The model under review builds one solid part; all positions refer to its coordinate system, in mm. Face numbers are marked on the shaded views. A direction names the side the tool comes from. Coordinates: 2 decimals unless noted, no trailing zeros. Loops run counter-clockwise (first coordinate to the right, second up) from the corner with the lowest first, then second, coordinate; pieces in that order, holes last. Notation, with made-up numbers: M 13,83 L 23,83 A32 ccw 23,115 Z; hole C 5,81 d7. An arc over 180 degrees is marked long. Use CSV: the item, a comma, the result in double quotes. Start each with the question number.
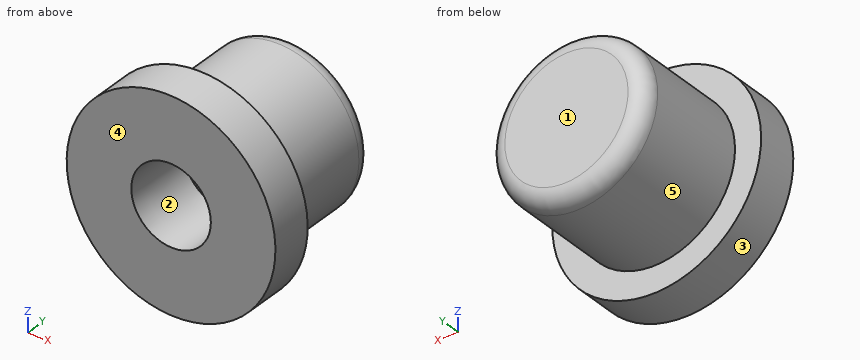
from build123d import *

# Parameters (mm, degrees)
EXTRUDE_1_DEPTH      = 3
EXTRUDE_1_DEPTH_BACK = 2.6
SKETCH_1_R           = 3.75
SKETCH_2_R           = 5
EXTRUDE_2_DEPTH      = 2
FILLET_1_R           = 0.8
SKETCH_3_R           = 1.905870149
SKETCH_4_R           = 1.852192046


# Read off the part's stored shape, not the designer's step: Отступ5
with BuildPart() as part:
    # Эскиз1 → Бобышка-Вытянуть1 (new, two sides: drawn at the far end of the back side and taken through both)
    with BuildSketch(Plane(origin=(0, 0, 0), x_dir=(1, 0, 0), z_dir=(0, 1, 0)).offset(-EXTRUDE_1_DEPTH_BACK)):
        with Locations(Location((0, 0, 0), (0, 0, 270))):
            Circle(SKETCH_1_R)
    extrude(amount=EXTRUDE_1_DEPTH + EXTRUDE_1_DEPTH_BACK)

    # Эскиз2 → Бобышка-Вытянуть2 (add)
    with BuildSketch(Plane.XZ.offset(2.6)):
        with Locations(Location((0, 0, 0), (0, 0, 270))):
            Circle(SKETCH_2_R)
    extrude(amount=EXTRUDE_2_DEPTH)

    # Скругление1
    fillet_1_edges = [part.edges().sort_by_distance(p)[0] for p in [
        (0, 3, -3.75),
    ]]
    fillet(fillet_1_edges, radius=FILLET_1_R)

    # Отступ5 outline → Отступ5 (revolve, cut)
    with BuildSketch(Plane.XY):
        with BuildLine():
            Line((1.605870149, -4.6), (1.552192046, -1.524783544))
            ThreePointArc((1.552192046, -1.524783544), (1.514226865, -1.436417193), (1.425211389, -1.4))
            Line((1.425211389, -1.4), (0, -1.4))
            Line((0, -1.4), (0, -4.6))
            Line((0, -4.6), (1.605870149, -4.6))
        make_face()
    revolve(axis=Axis((0, 0, 0), (0, 1, 0)), mode=Mode.SUBTRACT)

    # Эскиз3 → Вырез-По сечениям1 section 0
    with BuildSketch(Plane.XZ.offset(4.6)):
        Circle(SKETCH_3_R)
    # Эскиз4 → Вырез-По сечениям1 section 1
    with BuildSketch(Plane.XZ.offset(1.4)):
        Circle(SKETCH_4_R)
    loft(mode=Mode.SUBTRACT)


solid = part.part
1. For the marked faces 4 and 5, list the 3-axis set-ups (+Z, -Z, +X, -X, +Y, -Y) from which the entire face can be reached by the end or side of a thin tool; tool diameter is ignored.
2. Add section D-D (y = -3). Write out the cut boundary in (x, z), plus the area to 3 significant figures.
3. Add section B-B (z = 4). Write out the cut boundary in (x, y), plus the area to 3 significant figures.
4. Insertion check: pin 1 Ø4 at (y, z) = (1, -0.5) entering from -X; pin 2 Ø1.5 at (y, z) = (1, 2.5) entering from -X; pin 3 Ø1.1 at (x, z) = (0.5, 0) entering from -Y. Each pin has a flat end and moves straight along its axis. Give the tip position at first contact, or say it passes through.
5. Add section A-A (y = 0). Write out the cut boundary in (x, z), plus the area to 3 significant figures.
6. Add section C-C (y = -2). Write out the cut boundary in (x, z).
7. Draft analysis for pull direction X (two halves, no side actions). For the marked faces 1, 2 and 3, state which applies: released by +X, released by -X, zero draft, split by the parting line, or undercut.
8. To check wall thickness, follow line 1 along Y through (x, z) = (0.75, 1.25); line 2 along Y through (x, z) = (4.5, 0.5); line 3 along Z through (x, y) = (0.75, -1.5). State the ranges of each line that lie inside material, in increasing order.
Solved:
1,face 4,"+Z, -Z, +X, -X, -Y"
1,face 5,"+Y"
2,outline,"C 0,0 d10; hole C 0,0 d3.76"
2,area,"67.4 mm^2"
3,outline,"M -3,-4.6 L 3,-4.6 L 3,-2.6 L -3,-2.6 Z"
3,area,"12.0 mm^2"
4,pin 1,"stops at x = -3.75"
4,pin 2,"stops at x = -3.32"
4,pin 3,"stops at y = -1.4"
5,outline,"C 0,0 d7.5"
5,area,"44.2 mm^2"
6,outline,"C 0,0 d7.5; hole C 0,0 d3.72"
7,face 1,"zero draft"
7,face 2,"undercut"
7,face 3,"split by the parting line"
8,line 1,"y = -1.4 to 3"
8,line 2,"y = -4.6 to -2.6"
8,line 3,"z = -3.67 to -1.7, 1.7 to 3.67"
